Here's how the part is built. I have some questions about the finished solid (model axes, mm). A direction names the side the tool comes from. Give positions to 0.01 mm unless a question says otherwise; leave off trailing zeros. Write each loop counter-clockwise with the first axis right and the second up, starting at its lowest first coordinate (ties: lowest second). Pieces come first, ordered by that corner, then holes. Notation, with made-up numbers: (-27.75, 82.25) -> (15.25, 82.25) arc R33 cw to (15.25, 117.25) -> close; hole circle Ø7 at (21, 12). An arc over 180 degrees is marked (long way). Return JSON: item names as keys, results as strings.
Autodesk Inventor part; units mm, degrees
ref_plane "YZ Plane" through (0, 0, 0) normal (1, 0, 0) x (0, 1, 0)
ref_plane "XZ Plane" through (0, 0, 0) normal (0, 1, 0) x (-1, 0, 0)
ref_plane "XY Plane" through (0, 0, 0) normal (0, 0, 1) x (1, 0, 0)
sketch "Sketch1" plane through (0, 0, 0) normal (0, 0, 1) x (1, 0, 0)
  line L0 (0, -6.35) -> (25.4, -6.35)
  line L1 (25.4, -6.35) -> (25.4, -31.75)
  line L2 (25.4, -31.75) -> (-25.4, -31.75)
  line L3 (-25.4, -31.75) -> (-25.4, -6.35)
  line L4 (-25.4, -6.35) -> (0, -6.35)
  point P0 (-6.35, -6.35)
  point P1 (6.35, -6.35)
  dimension "d7" = 25.4
  dimension "d8" = 25.4
  dimension "d9" = 50.8
extrude "Extrusion1" add sketch "Sketch1" along normal blind 2
sketch "Sketch2" plane through (0, 0, 2) normal (0, 0, 1) x (1, 0, 0)
  line L0 (-25.4, -6.35) -> (-25.4, -31.75)
  line L1 (-25.4, -31.75) -> (7.1, -31.75)
  line L2 (-25.4, -31.75) -> (25.4, -31.75)
  line L3 (7.1, -31.75) -> (7.1, -30.75)
  line L4 (7.1, -30.75) -> (7.1, -28.75)
  circle A0 centre (7.1, -28.75) radius 2
  circle A1 centre (7.1, -9.35) radius 2
  line L5 (5.1, -9.35) -> (5.1, -28.75)
  line L6 (9.1, -9.35) -> (9.1, -28.75)
  point P0 (0, 0)
  dimension "d10" = 32.5
  dimension "d11" = 1
  dimension "d12" = 2
  dimension "d13" = 4
  dimension "d15" = 4
extrude "Extrusion2" cut sketch "Sketch2" against normal blind 2.54
sketch "Sketch3" plane through (0, 0, 0) normal (0, 0, 1) x (1, 0, 0)
  line L0 (-25.4, -6.35) -> (-25.4, -31.75)
  line L1 (-25.4, -6.35) -> (-25.4, -31.75)
  line L2 (-25.4, -31.75) -> (-35.4, -31.75)
  line L3 (-29.4, 26.95) -> (-35.4, 26.95)
  line L4 (-35.4, 26.95) -> (-35.4, -31.75)
  line L5 (-29.4, 26.95) -> (-25.4, 26.95)
  line L6 (-25.4, 26.95) -> (-25.4, -6.35)
  line L7 (25.4, -6.35) -> (-25.4, -6.35)
  line L8 (0, -6.35) -> (0, -31.75)
  line L9 (-25.4, -31.75) -> (25.4, -31.75)
  line L10 (25.4, -6.35) -> (25.4, -31.75)
  line L11 (25.4, -6.35) -> (25.4, -31.75)
  line L12 (25.4, -31.75) -> (35.4, -31.75)
  line L13 (29.4, 26.95) -> (35.4, 26.95)
  line L14 (35.4, 26.95) -> (35.4, -31.75)
  line L15 (29.4, 26.95) -> (25.4, 26.95)
  line L16 (25.4, 26.95) -> (25.4, -6.35)
  line L17 (-30.4, -31.75) -> (-30.4, -26.75)
  arc A0 (-32.525, -26.75) -> (-28.275, -26.75) centre (-30.4, -26.75) ccw
  line L18 (-30.4, 26.95) -> (-30.4, 21.95)
  arc A1 (-28.275, 21.95) -> (-32.525, 21.95) centre (-30.4, 21.95) ccw
  line L19 (-32.525, 21.95) -> (-32.525, -26.75)
  line L20 (-28.275, -26.75) -> (-28.275, 21.95)
  arc A2 (28.275, -26.75) -> (32.525, -26.75) centre (30.4, -26.75) ccw
  arc A3 (32.525, 21.95) -> (28.275, 21.95) centre (30.4, 21.95) ccw
  line L21 (32.525, 21.95) -> (32.525, -26.75)
  line L22 (28.275, -26.75) -> (28.275, 21.95)
  point P0 (0, 0)
  dimension "d26" = 10
  dimension "d36" = 5
  dimension "d37" = 4.25
  dimension "d38" = 5
  dimension "d39" = 4.25
extrude "Extrusion3" add sketch "Sketch3" along normal blind 2 contours L0 L2 L17 A0 L20 A1 L18 L3 L5 L6 | L2 L4 L3 L18 A1 L19 A0 L17 | L16 L15 L13 L14 L12 L10
fillet "Fillet1" radius 5 6 edges at (-35.4, 26.95, 1) (-25.4, 26.95, 1) (-35.4, -31.75, 1) (25.4, 26.95, 1) (35.4, 26.95, 1) (35.4, -31.75, 1)
properties part number "Ultrasonic Sensor"
1. Which directions (+Z, -Z, +X, -X, +Y, -Y) give clear straight access to the entire face, cutting with the end or side of a thin tool? Please do faces 1 (the face through (-30.447, 24.074, 0.986)), 2 (the face through (-33.9, 25.52, 1.01)), 3 (the face through (25.4, 8, 1)).
Taken from the geometry:
{"face 1": "+Z, -Z", "face 2": "+Z, -Z, -X, +Y", "face 3": "+Z, -Z, +Y"}
2. Suppose I cut it at A-A, the plane x = 7.1. List the corners of the cut face in (y, z) for me.
Taken from the geometry:
{"outline": "(-31.75, 0) -> (-30.75, 0) -> (-30.75, 2) -> (-31.75, 2) -> close; (-7.35, 0) -> (-6.35, 0) -> (-6.35, 2) -> (-7.35, 2) -> close"}
3. Suppose I cut it at C-C, the plane z = 1.15. Count the separate pieces of the cut face and the enclosed holes in it, and give its area (3 significant figures).
Taken from the geometry:
{"separate pieces": "1", "enclosed holes": "3", "area": "1,900 mm²"}
4. If we mould it in two halves opening along Y, with no side actions, what happens to faces 4 (the face through (33.97, 25.45, 1.01)), 5 (the face through (-35.4, -2, 1)), 6 (the face through (5.1, -19, 1)), 7 (the face through (30.447, -28.874, 0.986))? For each: released by +Y, released by -Y, zero draft, split by the parting line, or undercut.
Taken from the geometry:
{"face 4": "released by +Y", "face 5": "zero draft", "face 6": "undercut", "face 7": "undercut"}
5. If I drill on line 1 (X direction, y = 5.5, z = 0.2) (3 decimals); line 2 (X direction, y = -21, z = 0.1) (3 decimals); line 3 (Y direction, x = 7, z = 1.25), over which ranges is the centre line in solid material (lowest first)? Write a range as [from, to].
Taken from the geometry:
{"line 1": "x = [-35.4, -32.525], [-28.275, -25.4], [25.4, 28.275], [32.525, 35.4]", "line 2": "x = [-35.4, -32.525], [-28.275, 5.1], [9.1, 28.275], [32.525, 35.4]", "line 3": "y = [-31.75, -30.75], [-7.35, -6.35]"}
6. Suppose I cut it at B-B, the plane y = 14. List the corners of the cut face in (x, z) for me (3 decimals).
Taken from the geometry:
{"outline": "(-35.4, 0) -> (-32.525, 0) -> (-32.525, 2) -> (-35.4, 2) -> close; (-28.275, 0) -> (-25.4, 0) -> (-25.4, 2) -> (-28.275, 2) -> close; (25.4, 0) -> (28.275, 0) -> (28.275, 2) -> (25.4, 2) -> close; (32.525, 0) -> (35.4, 0) -> (35.4, 2) -> (32.525, 2) -> close"}
7. Suppose I cut it at D-D, the plane y = -21. List the corners of the cut face in (x, z) for me (3 decimals).
Taken from the geometry:
{"outline": "(-35.4, 0) -> (-32.525, 0) -> (-32.525, 2) -> (-35.4, 2) -> close; (-28.275, 0) -> (5.1, 0) -> (5.1, 2) -> (-28.275, 2) -> close; (9.1, 0) -> (28.275, 0) -> (28.275, 2) -> (9.1, 2) -> close; (32.525, 0) -> (35.4, 0) -> (35.4, 2) -> (32.525, 2) -> close"}
